from build123d import *

# Parameters (mm, degrees)
F0_R     = 1.6875
F0_R_2   = 2
F1_DEPTH = 56.5
F3_START = -4
F3_DEPTH = 48.5
F5_R     = 5
F6_R     = 2


# Not quite as in the source:
# - a feature of the source that left no trace in its solid (it failed there, or was rolled back) is left out
# - a feature names something its author has since deleted; it is built from what else it names


with BuildPart() as f1:
    # F0 (on Front) → F1 (new body)
    with BuildSketch(Plane.XZ):
        with BuildLine():
            ThreePointArc((-3.2424633134, -0.2212050215), (-1.5238508153, 2.8706059801), (2, 2.5617376915))
            Line((2, 2.5617376915), (2, 9.4382623085))
            ThreePointArc((2, 9.4382623085), (3.25, 12), (2, 14.5617376915))
            Line((2, 14.5617376915), (2, 16))
            Line((2, 16), (2, 26.0145742767))
            Line((2, 26.0145742767), (-1.3932364987, 38.9411094094))
            Line((-1.3932364987, 38.9411094094), (-1.8768517883, 38.8141596092))
            Line((-1.8768517883, 38.8141596092), (-1.5244873121, 39.4411094094))
            Line((-1.5244873121, 39.4411094094), (-1.6557381254, 39.9411094094))
            Line((-1.6557381254, 39.9411094094), (-2.1393534149, 39.8141596092))
            Line((-2.1393534149, 39.8141596092), (-1.7869889387, 40.4411094094))
            Line((-1.7869889387, 40.4411094094), (-1.918239752, 40.9411094094))
            Line((-1.918239752, 40.9411094094), (-2.4018550415, 40.8141596092))
            Line((-2.4018550415, 40.8141596092), (-2.0494905653, 41.4411094094))
            Line((-2.0494905653, 41.4411094094), (-2.1807413786, 41.9411094094))
            Line((-2.1807413786, 41.9411094094), (-2.6643566681, 41.8141596092))
            Line((-2.6643566681, 41.8141596092), (-2.3119921919, 42.4411094094))
            Line((-2.3119921919, 42.4411094094), (-2.4432430052, 42.9411094094))
            Line((-2.4432430052, 42.9411094094), (-6.0546269865, 41))
            Line((-6.0546269865, 41), (-3.2424633134, -0.2212050215))
        make_face()
        with Locations((0, 12)):
            Circle(F0_R, mode=Mode.SUBTRACT)
        with BuildLine():
            ThreePointArc((3.25, 0), (2.9208303614, 1.4252192814), (2, 2.5617376915))
            ThreePointArc((2, 2.5617376915), (-1.5238508153, 2.8706059801), (-3.2424633134, -0.2212050215))
            ThreePointArc((-3.2424633134, -0.2212050215), (0.1106666878, -3.2481152819), (3.25, 0))
        make_face()
        Circle(F0_R_2, mode=Mode.SUBTRACT)
        Circle(F0_R_2)
        Circle(F0_R, mode=Mode.SUBTRACT)
    extrude(amount=F1_DEPTH)

    # F2 (on face) → F3 (cut)
    with BuildSketch(Plane(origin=(0, 0, 0), x_dir=(-1, 0, 0), z_dir=(0, 1, 0)).offset(F3_START)):
        with BuildLine():
            Line((5.032301952, 26.0145742767), (-2, 26.0145742767))
            Line((-2, 26.0145742767), (-2.5801925668, 13.9761341853))
            ThreePointArc((-2.5801925668, 13.9761341853), (-3.2462320816, 12.1564521408), (-2.7582721639, 10.2811530987))
            Line((-2.7582721639, 10.2811530987), (-3.2462320816, 0.1564521408))
            ThreePointArc((-3.2462320816, 0.1564521408), (-0.1888379833, -3.2445092412), (3.2424633134, -0.2212050215))
            Line((3.2424633134, -0.2212050215), (5.032301952, 26.0145742767))
        make_face()
    extrude(amount=-F3_DEPTH, mode=Mode.SUBTRACT)

    # F5
    f5_edges = [f1.edges().sort_by_distance(p)[0] for p in [
        (2, -2, 9.438262),
        (2, -54.5, 9.438262),
        (2, -2, 2.561738),
        (2, -2, 14.561738),
        (2, -54.5, 14.561738),
        (2, -54.5, 2.561738),
    ]]
    fillet(f5_edges, radius=F5_R)

    # F6
    f6_edges = [f1.edges().sort_by_distance(p)[0] for p in [
        (-1.516151, -52.5, 26.014574),
        (-1.516151, -4, 26.014574),
    ]]
    fillet(f6_edges, radius=F6_R)


solid = f1.part
Verification items for the finished model (mm, model axes). A direction names the side the tool comes from. Give positions to 0.01 mm unless a question says otherwise; leave off trailing zeros. Order: outer loops, then holes, each group sorted by start corner. A loop starts at its lowest first (then second) coordinate and runs counter-clockwise, first axis right, second up. Notation, with made-up numbers: M -31,75 L 8,75 A21 cw 8,79 Z; hole C -4,-26 d3. An arc over 180 degrees is marked long. Use one line per item in the form item = value. Start each with the question number.
Q1. Section check C-C (z = 12). Enter the section's corners in (x, y).
Q2. Section check A-A (y = -29). Enter the section's corners in (x, z).
Q3. Go/stop test with flat-tipped pins: pin 1 Ø3.5 at (y, z) = (-1.5, 6) entering from +X; pin 2 Ø1 at (x, y) = (-4, -30.5) entering from -Z; pin 3 Ø2.5 at (x, z) = (0, 0) entering from -Y; pin 4 Ø2 at (x, z) = (-4.5, 20.5) entering from +Y. Record where each tip stops, or that it passes through.
Q4. Mould release check, pull along Y, two halves, no side actions. Record for faces 5 (the flat face through (-1, 0, 20)), 6 (the flat face through (-2, -4, 11)), 7 (the cylindrical face through (2.188, -2.028, 8.991)): +Y half, -Y half, draft (parallel to the pull), parting line (faces both ways), or undercut.
Q5. Scan lines: line 1 along Y through (x, z) = (1.5, 14); line 2 along X through (y, z) = (-54, 0); line 3 along Z through (x, y) = (-2.5, -7.5). Record each from-to range of solid material in increasing order. Write a range as [from, to].
Q6. Access from +Z, -Z, +X, -X, +Y, -Y to the whole of each face (thin tool, end or side, straight path). Record for faces 1 (the cylindrical face through (0.779, -1.972, 10.503)), 2 (the cylindrical face through (-1.467, -51.899, 25.444)), 3 (the flat face through (2, -2, 21)), 4 (the cylindrical face through (2.2, -2.03, 2.97)).
Q7. Section check B-B (x = 0). Enter the section's corners in (y, z).
Q8. Section check D-D (z = 22). Enter the section's corners in (x, y), then the cut area to 3 significant figures.
Evaluation:
q1.outline = M -4.08,-56.5 L -1.69,-56.5 L -1.69,-52.5 L -4.08,-52.5 Z; M -4.08,-4 L -1.69,-4 L -1.69,0 L -4.08,0 Z; M 1.69,-56.5 L 3.25,-56.5 L 3.25,-52.5 L 1.69,-52.5 Z; M 1.69,-4 L 3.25,-4 L 3.25,0 L 1.69,0 Z
q2.outline = M -6.05,41 L -5.03,26.01 L 2,26.01 L -1.39,38.94 L -1.88,38.81 L -1.52,39.44 L -1.66,39.94 L -2.14,39.81 L -1.79,40.44 L -1.92,40.94 L -2.4,40.81 L -2.05,41.44 L -2.18,41.94 L -2.66,41.81 L -2.31,42.44 L -2.44,42.94 Z
q3.pin_1 = 2
q3.pin_2 = 26.01
q3.pin_3 = through
q3.pin_4 = 0
q4.face_5 = +Y half
q4.face_6 = undercut
q4.face_7 = draft
q5.line_1 = [-56.5, -52.5], [-4, 0]
q5.line_2 = [-3.26, -1.69], [1.69, 3.25]
q5.line_3 = [26.01, 41.86], [42.11, 42.91]
q6.face_1 = +Y, -Y
q6.face_2 = -Z, +X, -X
q6.face_3 = +Z, +X, +Y, -Y
q6.face_4 = +X, +Y, -Y
q7.outline = M -56.5,-3.25 L -52.5,-3.25 L -52.5,-1.69 L -56.5,-1.69 Z; M -56.5,1.69 L -52.5,1.69 L -52.5,10.31 L -56.5,10.31 Z; M -56.5,13.69 L -52.5,13.69 L -52.5,24.01 A2 cw -50.5,26.01 L -6,26.01 A2 cw -4,24.01 L -4,13.69 L 0,13.69 L 0,33.63 L -56.5,33.63 Z; M -4,-3.25 L 0,-3.25 L 0,-1.69 L -4,-1.69 Z; M -4,1.69 L 0,1.69 L 0,10.31 L -4,10.31 Z
q8.outline = M -4.76,-56.5 L 2,-56.5 L 2,-52.5 L -4.76,-52.5 Z; M -4.76,-4 L 2,-4 L 2,0 L -4.76,0 Z
q8.area = 54.1 mm2
